```python
from build123d import *

# Parameters (mm, degrees)
SKETCH1_R                 = 150.00000000000003
SKETCH1_R_2               = 120
BOSS_EXTRUDE1_DEPTH       = 20
SKETCH2_R                 = 2.0000000000000018
CUT_EXTRUDE1_DEPTH        = 3.5
CIRPATTERN1_COUNT         = 3
SKETCH8_R                 = 150.00000000000006
SKETCH8_R_2               = 130
BOSS_EXTRUDE2_DEPTH       = 4
SPLIT1_SURFACE_1_BACK     = 425.942
SPLIT1_SURFACE_1_DEPTH    = 851.884
SPLIT1_SURFACE_2_BACK     = 425.942
SPLIT1_SURFACE_2_DEPTH    = 851.884
FILLET1_R                 = 15
SKETCH9_R                 = 2.049999999999871
BOSS_EXTRUDE3_DEPTH       = 24
FILLET2_R                 = 6
CIRPATTERN2_COUNT         = 3
FILLET2_OF_CIRPATTERN2_R  = 6
BOSS_EXTRUDE6_REACH       = 348.117
BOSS_EXTRUDE6_END_RADIUS  = 150.00000000000003
FILLET5_R                 = 8
M6X1_0_TAPPED_HOLE1_D     = 5
M6X1_0_TAPPED_HOLE1_DEPTH = 15
M6X1_0_TAPPED_HOLE1_TIP   = 1.5021515475689007


with BuildPart() as part:
    # Sketch1 → Boss-Extrude1 (new body)
    with BuildSketch(Plane.XY):
        Circle(SKETCH1_R)
        Circle(SKETCH1_R_2, mode=Mode.SUBTRACT)
    extrude(amount=BOSS_EXTRUDE1_DEPTH)

    # Sketch2 → Cut-Extrude1 (cut)
    with BuildSketch(Plane.XY.offset(20)):
        with Locations((0, 124)):
            Circle(SKETCH2_R)
    cut_extrude1 = extrude(amount=-CUT_EXTRUDE1_DEPTH, mode=Mode.SUBTRACT)

    # CirPattern1: Cut-Extrude1 ×3 about axis
    cirpattern1_axis = Axis((-4.94e-15, -7.48e-15, 0), (0, 0, 1))
    for i in range(1, CIRPATTERN1_COUNT):
        add(cut_extrude1.rotate(cirpattern1_axis, i * 360 / CIRPATTERN1_COUNT), mode=Mode.SUBTRACT)

    # Sketch8 → Boss-Extrude2 (add)
    with BuildSketch(Plane.XY.offset(20)):
        Circle(SKETCH8_R)
        Circle(SKETCH8_R_2, mode=Mode.SUBTRACT)
    extrude(amount=BOSS_EXTRUDE2_DEPTH)


with BuildPart() as body_2:
    # Split1: the piece behind the surface
    add(part.part)
    # Split1 surface: a surface, the sketch's curves swept straight by 851.884 mm
    with BuildLine(Plane.XY.offset(20).offset(-SPLIT1_SURFACE_1_BACK), mode=Mode.PRIVATE) as split1_surface_1_path:
        Line((-60.71743008822855, 137.16192505021607), (0, 0))
        Line((0, 0), (-121.16379943401968, 88.42699648134986))
    split1_surface_1 = Shell.extrude(split1_surface_1_path.wire(), (0 * SPLIT1_SURFACE_1_DEPTH, 0 * SPLIT1_SURFACE_1_DEPTH, 1 * SPLIT1_SURFACE_1_DEPTH))
    split(bisect_by=split1_surface_1, keep=Keep.BOTTOM)

    # Fillet1
    fillet1_edges = [body_2.edges().sort_by_distance(p)[0] for p in [
        (-94.14865229404315, 116.77341851301341, 24),
    ]]
    fillet(fillet1_edges, radius=FILLET1_R)


with BuildPart() as part_1:
    add(part.part)

    # Split1: split by a surface, the side it looks to stays
    # Split1 surface: a surface, the sketch's curves swept straight by 851.884 mm
    with BuildLine(Plane.XY.offset(20).offset(-SPLIT1_SURFACE_2_BACK), mode=Mode.PRIVATE) as split1_surface_2_path:
        Line((-60.71743008822855, 137.16192505021607), (0, 0))
        Line((0, 0), (-121.16379943401968, 88.42699648134986))
    split1_surface_2 = Shell.extrude(split1_surface_2_path.wire(), (0 * SPLIT1_SURFACE_2_DEPTH, 0 * SPLIT1_SURFACE_2_DEPTH, 1 * SPLIT1_SURFACE_2_DEPTH))
    split(bisect_by=split1_surface_2, keep=Keep.TOP)

    # Sketch6 → Cut-Revolve2 (revolve, cut)
    with BuildSketch(Plane(origin=(0, 0, 0), x_dir=(0, 0, 1), z_dir=(-0.914412833668107, -0.40478286725485696, 0))):
        with BuildLine():
            Line((24, 135.00000000000006), (24, 150.00000000000006))
            Line((24, 150.00000000000006), (9, 150.00000000000006))
            ThreePointArc((9.000000000000004, 150.00000000000006), (19.606601717798213, 145.60660171779824), (23.999999999999993, 135.00000000000003))
        make_face()
    cut_revolve2 = revolve(axis=Axis((-60.71743008822857, 137.1619250502161, 24), (0, 0, -1)), mode=Mode.SUBTRACT)

    # Mirror1: Cut-Revolve2 across plane
    add(cut_revolve2.mirror(Plane(origin=(0, 0, 0), x_dir=(0, 0, 1), z_dir=(-0.7784894567534315, -0.6276576819602762, 0))), mode=Mode.SUBTRACT)


with BuildPart() as body_2_1:
    add(body_2.part)

    # Combine1: union part
    add(part_1.part)

    # Sketch9 → Boss-Extrude3 (add)
    # profile 1 of 3: a face of its own
    with BuildSketch(Plane.XY.offset(24)):
        with BuildLine():
            ThreePointArc((-3.262499377045517, 149.96451612903218), (-5.966798192877617, 154.36966728986033), (-4.24264068711927, 159.2426406871193))
            Line((-4.242640687119266, 159.2426406871193), (-14.15461886744679, 149.33066250679175))
            ThreePointArc((-14.1546188674468, 149.33066250679167), (-8.714324103983273, 149.7466545716823), (-3.2624993770454083, 149.9645161290323))
        make_face()
    # profile 2 of 3: a face of its own
    with BuildSketch(Plane.XY.offset(24)):
        with BuildLine():
            Line((14.154618867446969, 149.3306625067917), (4.242640687119273, 159.24264068711932))
            ThreePointArc((4.242640687119273, 159.24264068711932), (5.543277195067717, 157.29610059419056), (6, 155.00000000000003))
            ThreePointArc((6, 155.00000000000003), (5.27138483997677, 152.13425369774941), (3.262499377045641, 149.96451612903223))
            ThreePointArc((3.262499377045714, 149.96451612903223), (8.714324103983444, 149.7466545716823), (14.154618867446963, 149.33066250679167))
        make_face()
    # profile 3 of 3: a face of its own
    with BuildSketch(Plane.XY.offset(24)):
        with BuildLine():
            ThreePointArc((4.242640687119273, 159.24264068711932), (-3.07e-15, 161), (-4.242640687119268, 159.2426406871193))
            ThreePointArc((-4.24264068711927, 159.2426406871193), (-5.966798192877617, 154.36966728986033), (-3.262499377045517, 149.96451612903218))
            ThreePointArc((-3.2624993770454083, 149.9645161290323), (1.4921e-13, 150), (3.262499377045714, 149.96451612903223))
            ThreePointArc((3.262499377045641, 149.96451612903223), (5.27138483997677, 152.13425369774941), (6, 155.00000000000003))
            ThreePointArc((6, 155.00000000000003), (5.543277195067717, 157.29610059419056), (4.242640687119273, 159.24264068711932))
        make_face()
        with Locations((1.388e-14, 155.00000000000003)):
            Circle(SKETCH9_R, mode=Mode.SUBTRACT)
    boss_extrude3 = extrude(amount=-BOSS_EXTRUDE3_DEPTH)

    # Fillet2
    fillet2_edges = [body_2_1.edges().sort_by_distance(p)[0] for p in [
        (-14.154618867446795, 149.33066250679173, 12),
        (14.154618867446967, 149.33066250679167, 12),
    ]]
    fillet(fillet2_edges, radius=FILLET2_R)

    # CirPattern2: Boss-Extrude3 ×3 about axis
    cirpattern2_axis = Axis((1.08e-15, -6.48e-15, 0), (0, 0, 1))
    for i in range(1, CIRPATTERN2_COUNT):
        add(boss_extrude3.rotate(cirpattern2_axis, i * 360 / CIRPATTERN2_COUNT))

    # Fillet2 of CirPattern2
    fillet2_of_cirpattern2_edges = [body_2_1.edges().sort_by_distance(p)[0] for p in [
        (-122.24683786111865, -86.9235907734913, 12),
        (-136.40145672856548, -62.40707173330022, 12),
        (136.4014567285654, -62.407071733300505, 12),
        (122.24683786111846, -86.92359077349151, 12),
    ]]
    fillet(fillet2_of_cirpattern2_edges, radius=FILLET2_OF_CIRPATTERN2_R)

    # Boss-Extrude6: up to this cylinder (the profile starts outside it)
    boss_extrude6_end = Plane(origin=(0, 0, 12), z_dir=(0, 0, -1)) * Cylinder(BOSS_EXTRUDE6_END_RADIUS, 997.2340000000002, mode=Mode.PRIVATE)
    # Sketch12 → Boss-Extrude6 (add, up to the surface)
    with BuildSketch(Plane(origin=(0, -150.00000000000003, 0), x_dir=(-1, 0, 0), z_dir=(0, -1, 0)), mode=Mode.PRIVATE) as boss_extrude6_sk1:
        Polygon((0, 0), (-40, -4.9e-15), (-40.00000000000001, -24), (0, -24), align=None)
    boss_extrude6_tool1 = extrude(boss_extrude6_sk1.sketch, amount=-BOSS_EXTRUDE6_REACH, mode=Mode.PRIVATE) - boss_extrude6_end
    add(boss_extrude6_tool1.solids().sort_by_distance((20, -150, 12))[0])
    # Sketch12 → Boss-Extrude6 (add, up to the surface)
    with BuildSketch(Plane(origin=(0, -150.00000000000003, 0), x_dir=(-1, 0, 0), z_dir=(0, -1, 0)), mode=Mode.PRIVATE) as boss_extrude6_sk2:
        Polygon((40, 0), (40.00000000000001, -24), (0, -24), (0, 0), align=None)
    boss_extrude6_tool2 = extrude(boss_extrude6_sk2.sketch, amount=-BOSS_EXTRUDE6_REACH, mode=Mode.PRIVATE) - boss_extrude6_end
    add(boss_extrude6_tool2.solids().sort_by_distance((-20, -150, 12))[0])

    # Fillet5
    # the kernel refuses this fillet: 8 mm, written as the material it adds along each edge
    with BuildSketch(Plane(origin=(40.00000000000015, -144.56832294800958, 24), x_dir=(0.9584597244138898, 0.2852279030467574, 0), z_dir=(0, 0, -1))) as fillet5_piece_1:
        with BuildLine():
            CenterArc((5.947542883110703, 7.998508324991874), FILLET5_R, 200.42971386414416, 68.4638241646868)
            Line((-1.5492658555665646, 5.2060436903559735), (-1.699202030340109, 5.1501943976632605))
            ThreePointArc((-1.699202030340109, 5.1501943976632605), (-0.9279864836895695, 2.5573853806904863), (-0.1533535559062191, -0.04563646448748021))
            Line((-0.1533535559062191, -0.04563646448748021), (0.00308963266655187, -0.15997016649984888))
            ThreePointArc((0.00308963266655187, -0.15997016649984888), (2.8965306248915494, -0.1320310935977963), (5.7899716171165965, -0.15997016649985063))
            Line((5.7899716171165965, -0.15997016649985063), (5.793061249783145, 1.4e-16))
        make_face()
    extrude(amount=24)
    with BuildSketch(Plane(origin=(-40.00000000000015, -144.56832294800958, 24), x_dir=(1.57e-14, -1, 0), z_dir=(0, 0, -1))) as fillet5_piece_2:
        with BuildLine():
            CenterArc((5.969842900063457, 7.98187806972569), FILLET5_R, 197.67893389575954, 68.46382416468674)
            Line((-1.652342712497161, 5.552415888979961), (-1.804786424748387, 5.503826645365045))
            ThreePointArc((-1.804786424748387, 5.503826645365045), (-0.9527178418323817, 2.738548992526119), (-0.1542062111445539, -0.04266666666667149))
            Line((-0.1542062111445539, -0.04266666666667149), (2.51e-15, -0.1599999999999966))
            ThreePointArc((2.51e-15, -0.1599999999999966), (2.7158385259952267, -0.16000000000009607), (5.420913735028992, -0.15963756139451152))
            Line((5.420913735028992, -0.15963756139451152), (5.431677051990448, 0))
        make_face()
    extrude(amount=24)

    # M6x1.0 Tapped Hole1
    with Locations(Plane(origin=(0, -150.00000000000003, 0), x_dir=(-1, 0, 0), z_dir=(0, -1, 0))):
        with Locations((-25, -12), (25, -12)):
            Hole(M6X1_0_TAPPED_HOLE1_D / 2, depth=M6X1_0_TAPPED_HOLE1_DEPTH)
            with Locations((0, 0, -(M6X1_0_TAPPED_HOLE1_DEPTH + M6X1_0_TAPPED_HOLE1_TIP / 2))):  # 118° drill point
                Cone(0, M6X1_0_TAPPED_HOLE1_D / 2, M6X1_0_TAPPED_HOLE1_TIP, mode=Mode.SUBTRACT)


solid = body_2_1.part
```
Design review of the part built by this model. Coordinates are the model's own, in mm. A direction names the side the tool comes from. Coordinates: 2 decimals unless noted, no trailing zeros. Write each loop counter-clockwise with the first axis right and the second up, starting at its lowest first coordinate (ties: lowest second). Pieces come first, ordered by that corner, then holes. Notation, with made-up numbers: M -20,21.5 L 11,21.5 A38 ccw 11,59.5 Z; hole C 47,14 d3. An arc over 180 degrees is marked long. Answer as a JSON object with one key per item and string values.
Item 1: Machinability: for faces 1 (the flat face through (138.513, -70.289, 12.168)), 2 (the cylindrical face through (-128.524, 19.535, 21.972)), 3 (the flat face through (122, -53, 24)), 4 (the flat face through (-138.47, -70.13, 12.17)), which of the approach directions +Z, -Z, +X, -X, +Y, -Y give a long, thin tool a straight path to every point of the face, cutting with its end or side? Answer none if there is none.
Outcome:
{"face 1": "+Z, -Z, +X", "face 2": "+Z", "face 3": "+Z, +X, -X, +Y, -Y", "face 4": "+Z, -Z, -X"}
Item 2: Wall thickness on probe 1 along Y at (x, z) = (0, 17.25); probe 2 along X at (y, z) = (0, 21.4); probe 3 along Z at (x, y) = (-25, -143): over which ranges is each line inside the solid? List them lowest first.
Outcome:
{"probe 1": "-150 to -120, 120 to 122, 126 to 152.95, 157.05 to 161", "probe 2": "-150 to -130, 130 to 150", "probe 3": "0 to 9.5, 14.5 to 24"}
Item 3: Add section A-A, the plane x = 56. Give the boundary of the cut face in (y, z).
Outcome:
{"outline": "M -139.15,0 L -106.13,0 L -106.13,20 L -117.32,20 L -117.32,24 L -139.15,24 Z; M 106.13,0 L 139.15,0 L 139.15,24 L 117.32,24 L 117.32,20 L 106.13,20 Z"}
Item 4: Insertion check: pin 1 Ø8 at (x, z) = (-33, 15.5) entering from +Y; pin 2 Ø2 at (x, y) = (-108, -62) entering from +Z; pin 3 Ø5 at (x, y) = (0, 124) entering from +Z; pin 4 Ø3.5 at (x, y) = (0, 155) entering from +Z. Each pin has a flat end and moves straight along its axis. Give the tip position at first contact, or say it passes through.
Outcome:
{"pin 1": "y = 147.17", "pin 2": "z = 16.5", "pin 3": "z = 20", "pin 4": "through"}
Item 5: Draft analysis for pull direction X (two halves, no side actions). For faces 5 (the flat face through (-1, -150, 12)), 6 (the cylindrical face through (-139.463, -80.443, 12.168)), 7 (the flat face through (38, -115, 20)), state which applies: pulls with the +X half, pulls with the -X half, needs draft (parallel to the pull), parting line crosses it, or undercut.
Outcome:
{"face 5": "needs draft", "face 6": "pulls with the -X half", "face 7": "undercut"}
Item 6: Add section B-B, the plane y = 57. Give the boundary of the cut face in (x, z).
Outcome:
{"outline": "M -138.75,0 L -105.6,0 L -105.6,20 L -116.84,20 L -116.84,24 L -138.75,24 Z; M 105.6,0 L 138.75,0 L 138.75,24 L 116.84,24 L 116.84,20 L 105.6,20 Z"}
